```python
from build123d import *

# Parameters (mm, degrees)
SKETCH1_W           = 170
SKETCH1_H           = 280
BOSS_EXTRUDE1_DEPTH = 6
SKETCH2_R           = 5
CUT_EXTRUDE1_DEPTH  = 6
SKETCH3_W           = 41.455389413
SKETCH3_H           = 172.5
CUT_EXTRUDE2_DEPTH  = 10
FILLET1_R           = 2
SKETCH4_R           = 26
CUT_EXTRUDE3_DEPTH  = 10


with BuildPart() as part:
    # Sketch1 → Boss-Extrude1 (new body)
    with BuildSketch(Plane(origin=(0, 0, 0), x_dir=(1, 0, 0), z_dir=(0, 1, 0))):
        Rectangle(SKETCH1_W, SKETCH1_H)
    extrude(amount=BOSS_EXTRUDE1_DEPTH)

    # Sketch2 → Cut-Extrude1 (cut)
    with BuildSketch(Plane(origin=(0, 6, 0), x_dir=(1, 0, 0), z_dir=(0, 1, 0))):
        with Locations(Location((-57.5, 120, 0), (0, 0, 270))):
            Circle(SKETCH2_R)
        with Locations(Location((57.5, 120, 0), (0, 0, 270))):
            Circle(SKETCH2_R)
        with Locations(Location((0, 13.7, 0), (0, 0, 270))):
            Circle(SKETCH2_R)
        with Locations(Location((-57.5, -120, 0), (0, 0, 270))):
            Circle(SKETCH2_R)
        with Locations(Location((57.5, -120, 0), (0, 0, 270))):
            Circle(SKETCH2_R)
        with Locations(Location((-42.5, -92.5, 0), (0, 0, 270))):
            Circle(SKETCH2_R)
        with Locations(Location((42.5, -92.5, 0), (0, 0, 270))):
            Circle(SKETCH2_R)
    extrude(amount=-CUT_EXTRUDE1_DEPTH, mode=Mode.SUBTRACT)

    # Sketch3 → Cut-Extrude2 (cut)
    with BuildSketch(Plane(origin=(0, 6, 0), x_dir=(1, 0, 0), z_dir=(0, 1, 0))):
        with Locations((-64.272305293, 18.75)):
            Rectangle(SKETCH3_W, SKETCH3_H)
    extrude(amount=-CUT_EXTRUDE2_DEPTH, mode=Mode.SUBTRACT)

    # Fillet1
    fillet1_edges = [part.edges().sort_by_distance(p)[0] for p in [
        (-43.544610587, 3, -105),
        (-43.544610587, 3, 67.5),
        (-85, 3, 67.5),
        (-85, 3, -105),
    ]]
    fillet(fillet1_edges, radius=FILLET1_R)

    # Sketch4 → Cut-Extrude3 (cut)
    with BuildSketch(Plane(origin=(0, 6, 0), x_dir=(1, 0, 0), z_dir=(0, 1, 0))):
        with Locations(Location((0, -48.8, 0), (0, 0, 270))):
            Circle(SKETCH4_R)
    extrude(amount=-CUT_EXTRUDE3_DEPTH, mode=Mode.SUBTRACT)


solid = part.part
```
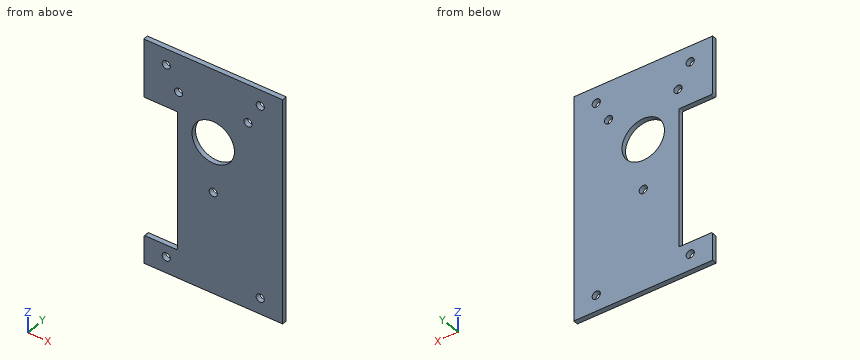
The listing builds one solid part. Answer for the finished solid, in the listing's coordinates (mm). Coordinates: 2 decimals unless noted, no trailing zeros. Loops run counter-clockwise (first coordinate to the right, second up) from the corner with the lowest first, then second, coordinate; pieces in that order, holes last. Notation, with made-up numbers: M -22,-10.75 L 32,-10.75 A20 ccw 32,15.25 Z; hole C -28,33 d8. An arc over 180 degrees is marked long. Answer as a JSON object with one key per item and string values. Group by question number.
Item 1: Section A-A (x = 0) is taken. Write down the section's boundary in (y, z).
Item 2: Consider L1, parallel to X at y = 2.9, z = -120; L2, parallel to X at y = 4.45, z = 92.5; L3, parallel to Z at x = -51, y = 1.75. Determine where each line is inside the solid, lowest interval first.
Item 3: Each of these flat-tipped pins is pushed along its axis until it touches: P1, Ø9, axis at x = -57.5, z = 120, coming from the -Y side; P2, Ø3, axis at y = 3, z = -29.5, coming from the -X side. Where does it stop, or does it pass through?
Item 4: Section C-C (z = 92.5) is taken. Write down the section's boundary in (x, y).
Item 5: Section B-B (z = -13.7) is taken. Write down the section's boundary in (x, y), and give its area (3 significant figures).
Item 6: Section D-D (x = 42.5) is taken. Write down the section's boundary in (y, z).
Solved:
{
 "1": {"outline": "M 0,-140 L 6,-140 L 6,-18.7 L 0,-18.7 Z; M 0,-8.7 L 6,-8.7 L 6,22.8 L 0,22.8 Z; M 0,74.8 L 6,74.8 L 6,140 L 0,140 Z"},
 "2": {"L1": "x = -85 to -62.5, -52.5 to 52.5, 62.5 to 85", "L2": "x = -85 to -47.5, -37.5 to 37.5, 47.5 to 85", "L3": "z = -140 to -105, 67.5 to 140"},
 "3": {"P1": "passes through", "P2": "stops at x = -43.54"},
 "4": {"outline": "M -85,0 L -47.5,0 L -47.5,6 L -85,6 Z; M -37.5,0 L 37.5,0 L 37.5,6 L -37.5,6 Z; M 47.5,0 L 85,0 L 85,6 L 47.5,6 Z"},
 "5": {"outline": "M -43.54,0 L -5,0 L -5,6 L -43.54,6 Z; M 5,0 L 85,0 L 85,6 L 5,6 Z", "area": "711 mm2"},
 "6": {"outline": "M 0,-140 L 6,-140 L 6,87.5 L 0,87.5 Z; M 0,97.5 L 6,97.5 L 6,140 L 0,140 Z"}
}
